Work out the finished part from the listing and answer in its coordinate system (mm). Face numbers are marked on the shaded views. Give positions to 0.01 mm unless a question says otherwise; leave off trailing zeros. Loops run counter-clockwise (first coordinate to the right, second up) from the corner with the lowest first, then second, coordinate; pieces in that order, holes last. Notation, with made-up numbers: (86.5, 2) -> (116.5, 2) arc R20 ccw to (116.5, 25) -> close; hole circle Ø11 at (-3.5, 69.25). An arc over 180 degrees is marked (long way). Answer as CSV lines item,"result". Start each with the question number.
1. Find section C-C, the plane x = 122. Give the vertices of the cut face in (y, z).
2. Find the intervals of material crossed by line 1 along Y through (x, z) = (-143.5, 4.5); line 2 along X through (y, z) = (64, 6.5); line 3 along X through (y, z) = (96, 12.5), in increasing order.
3. Find section A-A, the plane z = 22.5. Give the vertices of the cut face in (x, y), and give its area (3 significant figures).
4. Determine the mould class of the marked faces 1 and 2 for opening direction X: +X half, -X half, draft (parallel to the pull), parting line (faces both ways), or undercut.
5. Flat-ended cylindrical pins translate along their axes: pin 1 Ø8 at (y, z) = (14, 4.5) entering from +X; pin 2 Ø8 at (x, z) = (15.5, 4.5) entering from +Y; pin 3 Ø8 at (x, z) = (-20, 4.5) entering from -Y. Find the tip coordinate at first contact, or state that the pin passes through.
6. Find section B-B, the plane y = 42. Give the vertices of the cut face in (x, z).
7. Find section D-D, the plane x = 179.5. Give the vertices of the cut face in (y, z).
Autodesk Inventor part; units mm, degrees
ref_plane "YZ Plane" through (0, 0, 0) normal (1, 0, 0) x (0, 1, 0)
ref_plane "XZ Plane" through (0, 0, 0) normal (0, 1, 0) x (-1, 0, 0)
ref_plane "XY Plane" through (0, 0, 0) normal (0, 0, 1) x (1, 0, 0)
sketch "Sketch1" plane through (0, 0, 0) normal (0, 0, 1) x (1, 0, 0)
  line L0 (187.5, -112.5) -> (-187.5, -112.5)
  line L1 (-187.5, -112.5) -> (-187.5, 112.5)
  line L2 (-187.5, 112.5) -> (187.5, 112.5)
  line L3 (187.5, 112.5) -> (187.5, -112.5)
  line L4 (187.5, -112.5) -> (-187.5, 112.5) construction
  line L5 (-187.5, -112.5) -> (187.5, 112.5) construction
  line L6 (157.5, -83.3937) -> (-157.5, -83.3937)
  line L7 (-157.5, -83.3937) -> (-157.5, 83.3937)
  line L8 (-157.5, 83.3937) -> (157.5, 83.3937)
  line L9 (157.5, 83.3937) -> (157.5, -83.3937)
  line L10 (157.5, -83.3937) -> (-157.5, 83.3937) construction
  line L11 (-157.5, -83.3937) -> (157.5, 83.3937) construction
  point P0 (0, 0)
  dimension "d0" = 375
  dimension "d1" = 225
  dimension "d2" = 315
extrude "Extrusion1" add sketch "Sketch1" along normal blind 7.5
sketch "Sketch2" plane through (0, 0, 7.5) normal (0, 0, 1) x (1, 0, 0)
  line L0 (-157.5, 83.3937) -> (157.5, 83.3937)
  line L1 (-167.5, 83.3937) -> (-167.5, 118.3937)
  line L2 (-167.5, 118.3937) -> (-215.5, 118.3937)
  line L3 (-215.5, 118.3937) -> (-215.5, 83.3937)
  line L4 (-215.5, 83.3937) -> (-167.5, 83.3937)
  line L5 (167.5, 83.3937) -> (215.5, 83.3937)
  line L6 (215.5, 83.3937) -> (215.5, 118.3937)
  line L7 (215.5, 118.3937) -> (167.5, 118.3937)
  line L8 (167.5, 118.3937) -> (167.5, 83.3937)
  line L9 (157.5, -83.3937) -> (-157.5, -83.3937)
  line L10 (167.5, -83.3937) -> (215.5, -83.3937)
  line L11 (215.5, -83.3937) -> (215.5, -118.3937)
  line L12 (215.5, -118.3937) -> (167.5, -118.3937)
  line L13 (167.5, -118.3937) -> (167.5, -83.3937)
  line L14 (-167.5, -83.3937) -> (-215.5, -83.3937)
  line L15 (-215.5, -83.3937) -> (-215.5, -118.3937)
  line L16 (-215.5, -118.3937) -> (-167.5, -118.3937)
  line L17 (-167.5, -118.3937) -> (-167.5, -83.3937)
  point P0 (0, 0)
  dimension "d5" = 10
  dimension "d6" = 35
  dimension "d7" = 48
  dimension "d8" = 35
  dimension "d9" = 10
  dimension "d10" = 48
  dimension "d11" = 35
  dimension "d12" = 10
  dimension "d13" = 48
  dimension "d14" = 35
  dimension "d15" = 48
  dimension "d16" = 10
  dimension "d17" = 48
  dimension "d18" = 35
  dimension "d19" = 48
extrude "Extrusion2" add sketch "Sketch2" along normal blind 26
sketch "Sketch3" plane through (0, 0, 7.5) normal (0, 0, -1) x (-1, 0, 0)
  circle A0 centre (-203.5, 100.8937) radius 4
  line L0 (-187.5, -83.3937) -> (-215.5, -83.3937)
  line L1 (167.5, 118.3937) -> (215.5, 118.3937)
  line L2 (215.5, 118.3937) -> (215.5, 83.3937)
  circle A1 centre (-203.5, -100.8937) radius 4
  circle A2 centre (203.5, -100.8937) radius 4
  circle A3 centre (203.5, 100.8937) radius 4
  point P0 (0, 0)
  point P1 (-215.5, 118.3937)
  point P2 (215.5, -118.3937)
  dimension "d24" = 8
  dimension "d30" = 8
  dimension "d31" = 100.8937
  dimension "d32" = 203.5
  dimension "d33" = 203.5
  dimension "d34" = 100.8937
  dimension "d35" = 100.8937
  dimension "d36" = 203.5
  dimension "d37" = 100.8937
  dimension "d38" = 203.5
extrude "Extrusion3" add sketch "Sketch3" along normal blind 12
properties part number "RielesModificado"
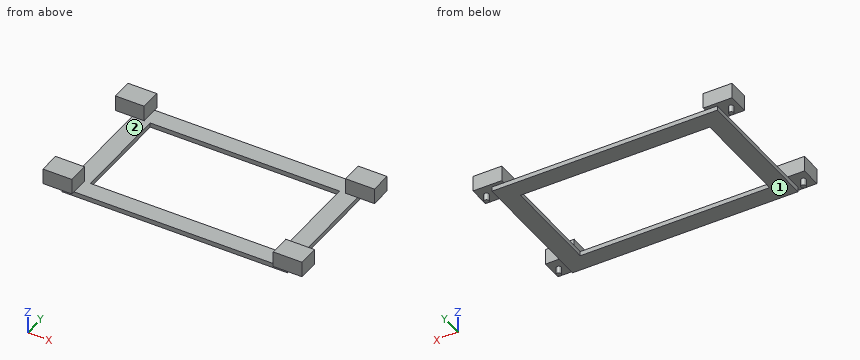
Resolved:
1,outline,"(-112.5, 0) -> (-83.39, 0) -> (-83.39, 7.5) -> (-112.5, 7.5) -> close; (83.39, 0) -> (112.5, 0) -> (112.5, 7.5) -> (83.39, 7.5) -> close"
2,line 1,"y = -112.5 to -83.39, 83.39 to 112.5"
2,line 2,"x = -187.5 to -157.5, 157.5 to 187.5"
2,line 3,"x = -215.5 to -167.5, 167.5 to 215.5"
3,outline,"(-215.5, -118.39) -> (-167.5, -118.39) -> (-167.5, -83.39) -> (-215.5, -83.39) -> close; (-215.5, 83.39) -> (-167.5, 83.39) -> (-167.5, 118.39) -> (-215.5, 118.39) -> close; (167.5, -118.39) -> (215.5, -118.39) -> (215.5, -83.39) -> (167.5, -83.39) -> close; (167.5, 83.39) -> (215.5, 83.39) -> (215.5, 118.39) -> (167.5, 118.39) -> close"
3,area,"6,720 mm^2"
4,face 1,"undercut"
4,face 2,"undercut"
5,pin 1,"stops at x = 187.5"
5,pin 2,"stops at y = 112.5"
5,pin 3,"stops at y = -112.5"
6,outline,"(-187.5, 0) -> (-157.5, 0) -> (-157.5, 7.5) -> (-187.5, 7.5) -> close; (157.5, 0) -> (187.5, 0) -> (187.5, 7.5) -> (157.5, 7.5) -> close"
7,outline,"(-118.39, 7.5) -> (-112.5, 7.5) -> (-112.5, 0) -> (112.5, 0) -> (112.5, 7.5) -> (118.39, 7.5) -> (118.39, 33.5) -> (83.39, 33.5) -> (83.39, 7.5) -> (-83.39, 7.5) -> (-83.39, 33.5) -> (-118.39, 33.5) -> close"
